Design review of the part built by this model. Coordinates are the model's own, in mm. A direction names the side the tool comes from. Round coordinates to 2 decimals unless told otherwise and drop trailing zeros. Order: outer loops, then holes, each group sorted by start corner. A loop starts at its lowest first (then second) coordinate and runs counter-clockwise, first axis right, second up. Notation, with made-up numbers: (45, -39.75) - (82, -39.75) arc R27 cw to (82, -12.75) - close; hole circle Ø11 at (68, -36). An arc over 180 degrees is marked (long way). Write item = value, one per line.
from build123d import *

# Parameters (mm, degrees)
SKETCH1_W           = 70
SKETCH1_H           = 40
BOSS_EXTRUDE1_DEPTH = 25
FILLET1_R           = 8
SHELL1_T            = -4
CHAMFER1_SIZE       = 10
CUT_EXTRUDE1_REACH  = 58.089
SKETCH2_R           = 11


with BuildPart() as part:
    # Sketch1 → Boss-Extrude1 (new, symmetric)
    with BuildSketch(Plane.XY):
        Rectangle(SKETCH1_W, SKETCH1_H)
    extrude(amount=BOSS_EXTRUDE1_DEPTH, both=True)

    # Fillet1
    fillet1_edges = [part.edges().sort_by_distance(p)[0] for p in [
        (35, -20, 0),
        (-35, -20, 0),
    ]]
    fillet(fillet1_edges, radius=FILLET1_R)

    # Shell1
    shell1_openings = [part.faces().sort_by_distance(p)[0] for p in [
        (0, 0.180447069, 25),
        (0, 0.180447069, -25),
        (0, 20, 0),
    ]]
    offset(amount=SHELL1_T, openings=shell1_openings, kind=Kind.INTERSECTION)

    # Chamfer1
    chamfer1_edges = [part.edges().sort_by_distance(p)[0] for p in [
        (-33, 20, -25),
        (-33, 20, 25),
        (33, 20, -25),
        (33, 20, 25),
    ]]
    chamfer(chamfer1_edges, length=CHAMFER1_SIZE)

    # Sketch2 → Cut-Extrude1 (cut, up to next)
    with BuildSketch(Plane(origin=(0, -16, 0), x_dir=(1, 0, 0), z_dir=(0, 1, 0)), mode=Mode.PRIVATE) as cut_extrude1_sk1:
        with Locations(Location((0, 0, 0), (0, 0, 270))):
            Circle(SKETCH2_R)
    cut_extrude1_tool1 = extrude(cut_extrude1_sk1.sketch, amount=-CUT_EXTRUDE1_REACH, mode=Mode.PRIVATE) & part.part
    add(cut_extrude1_tool1.solids().sort_by_distance((0, -16, 0))[0], mode=Mode.SUBTRACT)


solid = part.part
1) We need section D-D on z = -13. Write out the cut boundary in (x, y).
Findings:
outline = (-35, -12) arc R8 ccw to (-27, -20) - (27, -20) arc R8 ccw to (35, -12) - (35, 20) - (31, 20) - (31, -12) arc R4 cw to (27, -16) - (-27, -16) arc R4 cw to (-31, -12) - (-31, 20) - (-35, 20) - close
2) The part is to be moulded in two halves that separate along X. For faces 3 (the flat face through (-35, 4, 0)), 4 (the cylindrical face through (29.859, -14.797, 0.35)), 5 (the flat face through (-33, 20, 0)), say which applies: released by +X, released by -X, zero draft, split by the parting line, or undercut.
Findings:
face_3 = released by -X
face_4 = undercut
face_5 = zero draft
3) Clearance check with a flat-ended pin moving along its axis: pin 1 Ø1.5 at (x, z) = (25, 18) entering from +Y. State where the tip first meets the part, or that it passes through.
Findings:
pin_1 = -16
4) For faces 1 (the flat face through (31, 4, 0)), 2 (the flat face through (-33, 15, 20)), list the 3-axis set-ups (+Z, -Z, +X, -X, +Y, -Y) from which the entire face can be reached by the end or side of a thin tool; tool diameter is ignored.
Findings:
face_1 = +Z, -Z, +Y
face_2 = +Z, +X, -X, +Y
5) We need section C-C on y = 11. Write out the cut boundary in (x, z), and give its area (3 significant figures).
Findings:
outline = (-35, -24) - (-31, -24) - (-31, 24) - (-35, 24) - close; (31, -24) - (35, -24) - (35, 24) - (31, 24) - close
area = 384 mm^2
6) We need section B-B on x = 0. Write out the cut boundary in (y, z), and give its area (3 significant figures).
Findings:
outline = (-20, -25) - (-16, -25) - (-16, -11) - (-20, -11) - close; (-20, 11) - (-16, 11) - (-16, 25) - (-20, 25) - close
area = 112 mm^2
7) We need section A-A on z = 0. Write out the cut boundary in (x, y).
Findings:
outline = (-35, -12) arc R8 ccw to (-27, -20) - (-11, -20) - (-11, -16) - (-27, -16) arc R4 cw to (-31, -12) - (-31, 20) - (-35, 20) - close; (11, -20) - (27, -20) arc R8 ccw to (35, -12) - (35, 20) - (31, 20) - (31, -12) arc R4 cw to (27, -16) - (11, -16) - close
8) To check wall thickness, follow L1, parallel to X at y = -6.5, z = -12; L2, parallel to Y at x = -21, z = 0; L3, parallel to X at y = -17.9, z = 0. State the ranges of each line that lie inside material, in increasing order. Write a range as from..to.
Findings:
L1 = -35..-31, 31..35
L2 = -20..-16
L3 = -32.4..-11, 11..32.4
